from build123d import *

# Parameters (mm, degrees)
SKETCH1_W           = 152.4
SKETCH1_H           = 152.4
BOSS_EXTRUDE1_DEPTH = 101.6
SKETCH2_W           = 25.4
SKETCH2_H           = 19.05
BOSS_EXTRUDE2_DEPTH = 6.35
SKETCH3_W           = 139.7
SKETCH3_H           = 139.7
CUT_EXTRUDE1_DEPTH  = 95.25
FILLET1_R           = 9.652
CHAMFER1_SIZE       = 6.35
SKETCH4_R           = 3.81
CUT_EXTRUDE2_DEPTH  = 171.275704178
FILLET2_R           = 3.81
SKETCH5_R           = 6.35
BOSS_EXTRUDE3_DEPTH = 19.05
BOSS_EXTRUDE4_DEPTH = 95.25
SKETCH6_R           = 3.81
CUT_EXTRUDE3_DEPTH  = 17.272
CUT_EXTRUDE4_REACH  = 210.646
SKETCH8_R           = 12.7
CUT_EXTRUDE5_REACH  = 226.792
SKETCH9_R           = 12.7


with BuildPart() as part:
    # Sketch1 → Boss-Extrude1 (new body)
    with BuildSketch(Plane(origin=(0, 0, 0), x_dir=(1, 0, 0), z_dir=(0, 1, 0))):
        with Locations((2.134713764, -23.481851401)):
            Rectangle(SKETCH1_W, SKETCH1_H)
    extrude(amount=BOSS_EXTRUDE1_DEPTH)

    # Sketch2 → Boss-Extrude2 (add)
    with BuildSketch(Plane(origin=(0, 0, 0), x_dir=(1, 0, 0), z_dir=(0, 1, 0))):
        with Locations((87.224713764, -64.756851401)):
            Rectangle(SKETCH2_W, SKETCH2_H)
        with Locations((-82.955286236, -64.756851401)):
            Rectangle(SKETCH2_W, SKETCH2_H)
        with Locations((87.224713764, 17.793148599)):
            Rectangle(SKETCH2_W, SKETCH2_H)
        with Locations((-82.955286236, 17.793148599)):
            Rectangle(SKETCH2_W, SKETCH2_H)
    extrude(amount=BOSS_EXTRUDE2_DEPTH)

    # Sketch3 → Cut-Extrude1 (cut)
    with BuildSketch(Plane(origin=(0, 101.6, 0), x_dir=(1, 0, 0), z_dir=(0, 1, 0))):
        with Locations((2.134713764, -23.481851401)):
            Rectangle(SKETCH3_W, SKETCH3_H)
    extrude(amount=-CUT_EXTRUDE1_DEPTH, mode=Mode.SUBTRACT)

    # Fillet1
    # the kernel refuses this fillet: 9.652 mm, written as the material it takes off along each edge
    with BuildSketch(Plane(origin=(-95.655286236, -24.13, -27.318148599), x_dir=(1, 0, 0), z_dir=(0, 1, 0)), Plane(origin=(-95.655286236, -24.13, 55.231851401), x_dir=(1, 0, 0), z_dir=(0, 1, 0)), Plane(origin=(99.924713764, -24.13, -8.268148599), x_dir=(-1, 0, 0), z_dir=(0, 1, 0)), Plane(origin=(99.924713764, -24.13, 74.281851401), x_dir=(-1, 0, 0), z_dir=(0, 1, 0))) as fillet1_piece_1:
        with BuildLine():
            CenterArc((FILLET1_R, -FILLET1_R), FILLET1_R, 90, 90)
            Line((0, -FILLET1_R), (0, 0))
            Line((0, 0), (FILLET1_R, 0))
        make_face()
    extrude(amount=54.61, mode=Mode.SUBTRACT)
    with BuildSketch(Plane(origin=(-95.655286236, -24.13, -8.268148599), x_dir=(1, 0, 0), z_dir=(0, 1, 0)), Plane(origin=(-95.655286236, -24.13, 74.281851401), x_dir=(1, 0, 0), z_dir=(0, 1, 0)), Plane(origin=(99.924713764, -24.13, -27.318148599), x_dir=(-1, 0, 0), z_dir=(0, 1, 0)), Plane(origin=(99.924713764, -24.13, 55.231851401), x_dir=(-1, 0, 0), z_dir=(0, 1, 0))) as fillet1_piece_2:
        with BuildLine():
            CenterArc((FILLET1_R, FILLET1_R), FILLET1_R, 180, 90)
            Line((0, FILLET1_R), (0, 0))
            Line((0, 0), (FILLET1_R, 0))
        make_face()
    extrude(amount=54.61, mode=Mode.SUBTRACT)

    # Chamfer1
    chamfer1_edges = [part.edges().sort_by_distance(p)[0] for p in [
        (-74.065286236, 50.8, -52.718148599),
        (78.334713764, 50.8, -52.718148599),
        (78.334713764, 50.8, 99.681851401),
        (-74.065286236, 50.8, 99.681851401),
    ]]
    chamfer(chamfer1_edges, length=CHAMFER1_SIZE)

    # Sketch4 → Cut-Extrude2 (cut, through all)
    with BuildSketch(Plane(origin=(0, 6.35, 0), x_dir=(1, 0, 0), z_dir=(0, 1, 0))):
        with Locations(Location((90.272713764, -64.883851401, 0), (0, 0, 270))):
            Circle(SKETCH4_R)
        with Locations(Location((-86.003286236, -64.883851401, 0), (0, 0, 90))):
            Circle(SKETCH4_R)
        with Locations(Location((90.272713764, 17.920148599, 0), (0, 0, 90))):
            Circle(SKETCH4_R)
        with Locations(Location((-86.003286236, 17.920148599, 0), (0, 0, 270))):
            Circle(SKETCH4_R)
    extrude(amount=-CUT_EXTRUDE2_DEPTH, mode=Mode.SUBTRACT)

    # Fillet2
    fillet2_edges = [part.edges().sort_by_distance(p)[0] for p in [
        (-70.890286236, 0, 96.506851401),
        (-74.065286236, 0, 23.481851401),
        (-70.890286236, 0, -49.543148599),
        (2.134713764, 0, -52.718148599),
        (75.159713764, 0, -49.543148599),
        (78.334713764, 0, 23.481851401),
        (75.159713764, 0, 96.506851401),
        (2.134713764, 0, 99.681851401),
    ]]
    fillet(fillet2_edges, radius=FILLET2_R)

    # Sketch5 → Boss-Extrude3 (add)
    with BuildSketch(Plane(origin=(0, 101.6, 0), x_dir=(1, 0, 0), z_dir=(0, 1, 0))):
        with Locations((71.984713764, -93.331851401)):
            Circle(SKETCH5_R)
        with Locations((-67.715286236, -93.331851401)):
            Circle(SKETCH5_R)
        with Locations((-67.715286236, 46.368148599)):
            Circle(SKETCH5_R)
        with Locations((71.984713764, 46.368148599)):
            Circle(SKETCH5_R)
    extrude(amount=-BOSS_EXTRUDE3_DEPTH)

    # Sketch7 → Boss-Extrude4 (add)
    with BuildSketch(Plane(origin=(0, 101.6, 0), x_dir=(1, 0, 0), z_dir=(0, 1, 0))):
        with BuildLine():
            Line((71.984713764, -99.681851401), (78.334713764, -93.331851401))
            ThreePointArc((78.334713764, -93.331851401), (67.494585703, -88.84172334), (71.984713764, -99.681851401))
        make_face()
        with BuildLine():
            Line((-67.715286236, -99.681851401), (-74.065286236, -93.331851401))
            ThreePointArc((-74.065286236, -93.331851401), (-63.225158176, -88.84172334), (-67.715286236, -99.681851401))
        make_face()
        with BuildLine():
            Line((71.984713764, 52.718148599), (78.334713764, 46.368148599))
            ThreePointArc((78.334713764, 46.368148599), (67.494585703, 41.878020539), (71.984713764, 52.718148599))
        make_face()
        with BuildLine():
            Line((-67.715286236, 52.718148599), (-74.065286236, 46.368148599))
            ThreePointArc((-74.065286236, 46.368148599), (-63.225158176, 41.878020539), (-67.715286236, 52.718148599))
        make_face()
    extrude(amount=-BOSS_EXTRUDE4_DEPTH)

    # Sketch6 → Cut-Extrude3 (cut)
    with BuildSketch(Plane(origin=(0, 101.6, 0), x_dir=(1, 0, 0), z_dir=(0, 1, 0))):
        with Locations(Location((71.984713764, -93.331851401, 0), (0, 0, 270))):
            Circle(SKETCH6_R)
        with Locations(Location((-67.715286236, -93.331851401, 0), (0, 0, 90))):
            Circle(SKETCH6_R)
        with Locations(Location((71.984713764, 46.368148599, 0), (0, 0, 90))):
            Circle(SKETCH6_R)
        with Locations(Location((-67.715286236, 46.368148599, 0), (0, 0, 270))):
            Circle(SKETCH6_R)
    extrude(amount=-CUT_EXTRUDE3_DEPTH, mode=Mode.SUBTRACT)

    # Sketch8 → Cut-Extrude4 (cut, up to next)
    with BuildSketch(Plane.XY.offset(99.681851401), mode=Mode.PRIVATE) as cut_extrude4_sk1:
        with Locations((2.134713764, 52.705)):
            Circle(SKETCH8_R)
    cut_extrude4_tool1 = extrude(cut_extrude4_sk1.sketch, amount=-CUT_EXTRUDE4_REACH, mode=Mode.PRIVATE) & part.part
    add(cut_extrude4_tool1.solids().sort_by_distance((2.134714, 52.705, 99.681851))[0], mode=Mode.SUBTRACT)

    # Sketch9 → Cut-Extrude5 (cut, up to next)
    with BuildSketch(Plane.ZY.offset(74.065286236), mode=Mode.PRIVATE) as cut_extrude5_sk1:
        with Locations((23.481851401, 52.705)):
            Circle(SKETCH9_R)
    cut_extrude5_tool1 = extrude(cut_extrude5_sk1.sketch, amount=-CUT_EXTRUDE5_REACH, mode=Mode.PRIVATE) & part.part
    add(cut_extrude5_tool1.solids().sort_by_distance((-74.065286, 52.705, 23.481851))[0], mode=Mode.SUBTRACT)


solid = part.part
Work out the finished part from the listing and answer in its coordinate system (mm). A direction names the side the tool comes from. Coordinates: 2 decimals unless noted, no trailing zeros. Order: outer loops, then holes, each group sorted by start corner. A loop starts at its lowest first (then second) coordinate and runs counter-clockwise, first axis right, second up. Notation, with made-up numbers: (-39.5, 46.25) - (-1.5, 46.25) arc R20 cw to (-1.5, 64.25) - close; hole circle Ø1 at (49, -9). An arc over 180 degrees is marked (long way). Put each result on its own line as item: value. Start each with the question number.
1) Find section C-C (y = 15.5). Give the vertices of the cut face in (x, z).
2) Find the intervals of material crossed by line 1 (X direction, y = 85, z = 81.5); line 2 (Z direction, x = -44, y = 93); line 3 (Y direction, x = 4.5, z = -42.5), in increasing order. Write a range as from..to.
3) Find section D-D (z = -36.5). Give the vertices of the cut face in (x, y).
4) Find section A-A (y = 87.5). Give the vertices of the cut face in (x, z).
5) For faces 5 (the flat face through (75.204, 42.629, -49.499)), 6 (the cylindrical face through (97.13, 3.13, 58.09)), 7 (the flat face through (71.985, 55, 24)), determine the directions among +Z, -Z, +X, -X, +Y, -Y from which every point of the face is accessible in a straight line to the end or side of a thin tool.
6) For a pull along Z with two mould halves and no side action, classify faces 1 (the cylindrical face through (-70.359, 1.086, -48.454)), 2 (the flat face through (-13, 55, 93.332)), 3 (the cylindrical face through (-64.335, 93.085, 91.574)), 4 (the flat face through (-4, 101.6, 97)) as released by +Z, released by -Z, zero draft, split by the parting line, or undercut.
7) Flat-ended cylindrical pins translate along their axes: pin 1 (2.5 mm diameter, centred on x = -66.5, z = 93, fed in from +Y); pin 2 (7 mm diameter, centred on x = 82, y = 3, fed in from -Z); pin 3 (5 mm diameter, centred on x = -72.5, z = -50.5, fed in from -Y); pin 4 (21 mm diameter, centred on x = 87.5, z = 65.5, fed in from +Y). Find the tip coordinate at first contact, or state that the pin passes through.
8) Find section B-B (x = 50.5). Give the vertices of the cut face in (y, z).
Results list:
1. outline: (-74.07, -46.37) - (-67.72, -52.72) - (71.98, -52.72) - (78.33, -46.37) - (78.33, 93.33) - (71.98, 99.68) - (-67.72, 99.68) - (-74.07, 93.33) - close; hole (-67.72, -40.02) arc R6.35 cw to (-61.37, -46.37) - (65.63, -46.37) arc R6.35 cw to (71.98, -40.02) - (71.98, 86.98) arc R6.35 cw to (65.63, 93.33) - (-61.37, 93.33) arc R6.35 cw to (-67.72, 86.98) - close
2. line 1: x = -74.07..-67.72, 71.98..78.33
2. line 2: z = -52.72..-46.37, 93.33..99.68
2. line 3: y = 0..6.35
3. outline: (-74.07, 0) - (78.33, 0) - (78.33, 101.6) - (71.98, 101.6) - (71.98, 6.35) - (-67.72, 6.35) - (-67.72, 101.6) - (-74.07, 101.6) - close
4. outline: (-74.07, -46.37) arc R6.35 ccw to (-67.72, -52.72) - (71.98, -52.72) arc R6.35 ccw to (78.33, -46.37) - (78.33, 93.33) arc R6.35 ccw to (71.98, 99.68) - (-67.72, 99.68) arc R6.35 ccw to (-74.07, 93.33) - close; hole circle Ø7.62 at (-67.72, -46.37); hole circle Ø7.62 at (-67.72, 93.33); hole (-67.72, -40.02) arc R6.35 cw to (-61.37, -46.37) - (65.63, -46.37) arc R6.35 cw to (71.98, -40.02) - (71.98, 86.98) arc R6.35 cw to (65.63, 93.33) - (-61.37, 93.33) arc R6.35 cw to (-67.72, 86.98) - close; hole circle Ø7.62 at (71.98, -46.37); hole circle Ø7.62 at (71.98, 93.33)
5. face 5: -Z, +X, -Y
5. face 6: +X, +Y, -Y
5. face 7: +Y
6. face 1: released by -Z
6. face 2: undercut
6. face 3: undercut
6. face 4: zero draft
7. pin 1: stops at y = 84.33
7. pin 2: stops at z = -27.32
7. pin 3: stops at y = 1.63
7. pin 4: stops at y = 101.6
8. outline: (0, -48.91) arc R3.81 ccw to (3.81, -52.72) - (101.6, -52.72) - (101.6, -46.37) - (6.35, -46.37) - (6.35, 93.33) - (101.6, 93.33) - (101.6, 99.68) - (3.81, 99.68) arc R3.81 ccw to (0, 95.87) - close
